Input: part model. Units: mm. Frame: model coordinates. A direction names the side the tool comes from. Give positions to 0.01 mm unless a question says otherwise; leave off trailing zeros. Write each loop counter-clockwise with the first axis right and the second up, starting at its lowest first coordinate (ties: lowest second). Pieces come first, ordered by that corner, then holes. Notation, with made-up numbers: (76.25, 45.25) -> (80.25, 45.25) arc R9 cw to (80.25, 61.25) -> close; hole circle Ø5 at (31, 42.5). An arc over 180 degrees is marked (long way). Return JSON: item names as keys, results as strings. Group by question number.
Item 1: Section D-D, the plane x = -87.5. Return loops of the section in (y, z), then the cut area to 3 significant figures.
Item 2: Line query: line 1 (Y direction, x = -15, z = 1.9); line 2 (Z direction, x = -73.5, y = 11.5); line 3 (X direction, y = 12.25, z = 8.5). Output: solid intervals per line, ascending. Write a range as [from, to].
Item 3: Section A-A, the plane y = 12.5. Return loops of the section in (x, z).
Item 4: Section C-C, the plane y = 16.5. Return loops of the section in (x, z), then the cut area to 3 significant figures.
Item 5: Mould query, pull axis Y, two halves, no side actions, for faces 1 (the face through (-18.685, 15.879, 2.465)), 2 (the face through (-51, 25, 2)), 3 (the face through (-51, 13, 5)). Classes: released by +Y, released by -Y, zero draft, split by the parting line, or undercut.
Item 6: Pin query (flat end, axial travel): P1, Ø2, axis at x = -80, z = 13.5, coming from the +Y side; P2, Ø4, axis at x = -18, y = 21.5, coming from the +Z side. Return the tip coordinate at first contact, or that it passes through.
Item 7: Section B-B, the plane x = -15. Return loops of the section in (y, z), then the cut area to 3 significant figures.
Item 8: Set-up query: faces 4 (the face through (-88, 13, 15)), 5 (the face through (-82.881, 10.585, 9.93)). Return all of +Z, -Z, +X, -X, +Y, -Y with unobstructed straight access to the full face (end or side cutting, diameter ignored); none if empty.
from build123d import *

# Parameters (mm, degrees)
SKETCH1_W           = 100
SKETCH1_H           = 25
SKETCH1_R           = 5
BOSS_EXTRUDE1_DEPTH = 5
SKETCH2_R           = 5
BOSS_EXTRUDE2_DEPTH = 10


with BuildPart() as part:
    # Sketch1 → Boss-Extrude1 (new body)
    with BuildSketch(Plane.XY):
        with Locations((-50, 12.5)):
            Rectangle(SKETCH1_W, SKETCH1_H)
        with Locations((-15, 12.5)):
            Circle(SKETCH1_R, mode=Mode.SUBTRACT)
    extrude(amount=BOSS_EXTRUDE1_DEPTH)

    # Sketch2 → Boss-Extrude2 (add)
    with BuildSketch(Plane.XY.offset(5)):
        with Locations((-87.5, 12.5)):
            Circle(SKETCH2_R)
    extrude(amount=BOSS_EXTRUDE2_DEPTH)


solid = part.part
Answer below:
{
 "1": {"outline": "(0, 0) -> (25, 0) -> (25, 5) -> (17.5, 5) -> (17.5, 15) -> (7.5, 15) -> (7.5, 5) -> (0, 5) -> close", "area": "225 mm2"},
 "2": {"line 1": "y = [0, 7.5], [17.5, 25]", "line 2": "z = [0, 5]", "line 3": "x = [-92.49, -82.51]"},
 "3": {"outline": "(-100, 0) -> (-20, 0) -> (-20, 5) -> (-82.5, 5) -> (-82.5, 15) -> (-92.5, 15) -> (-92.5, 5) -> (-100, 5) -> close; (-10, 0) -> (0, 0) -> (0, 5) -> (-10, 5) -> close"},
 "4": {"outline": "(-100, 0) -> (-18, 0) -> (-18, 5) -> (-84.5, 5) -> (-84.5, 15) -> (-90.5, 15) -> (-90.5, 5) -> (-100, 5) -> close; (-12, 0) -> (0, 0) -> (0, 5) -> (-12, 5) -> close", "area": "530 mm2"},
 "5": {"face 1": "undercut", "face 2": "released by +Y", "face 3": "zero draft"},
 "6": {"P1": "passes through", "P2": "stops at z = 5"},
 "7": {"outline": "(0, 0) -> (7.5, 0) -> (7.5, 5) -> (0, 5) -> close; (17.5, 0) -> (25, 0) -> (25, 5) -> (17.5, 5) -> close", "area": "75.0 mm2"},
 "8": {"face 4": "+Z, +X, -X, +Y, -Y", "face 5": "+Z"}
}
